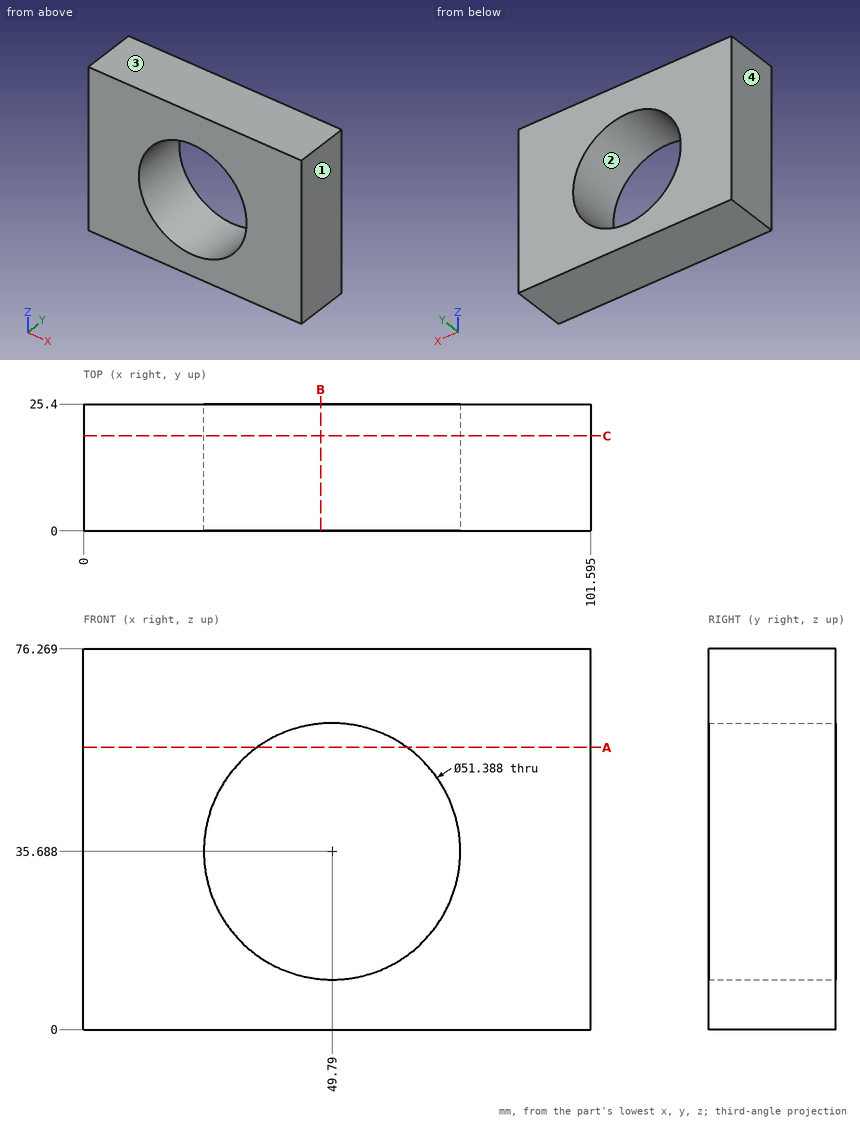
Answer from the drawing. Dimensions are ordinates in mm from the lowest x, y and z of the part. Coordinates: 2 decimals unless noted, no trailing zeros. Order: outer loops, then holes, each group sorted by start corner. A loop starts at its lowest first (then second) coordinate and runs counter-clockwise, first axis right, second up. Notation, with made-up numbers: (67.5, -1.5) -> (108.5, -1.5) arc R22 ccw to (108.5, 20.5) -> close; hole circle Ø8 at (74, 51). An arc over 180 degrees is marked (long way). Answer as a JSON object with one key per item and string values.
1) This flat-tipped pin is pushed along its axis until it touches: pin 1 (4 mm diameter, centred on x = 68, z = 22, fed in from -Y). Where does it stop, or does it pass through?
Model answer:
{"pin 1": "passes through"}
2) A cutting plane is placed at B-B, the plane x = 47.5. Determine the outline of the cut face in (y, z).
Model answer:
{"outline": "(0, 0) -> (25.4, 0) -> (25.4, 10.1) -> (0, 10.1) -> close; (0, 61.28) -> (25.4, 61.28) -> (25.4, 76.27) -> (0, 76.27) -> close"}
3) A cutting plane is placed at C-C, the plane y = 19. Determine the outline of the cut face in (x, z) (1 decimal).
Model answer:
{"outline": "(0, 0) -> (101.6, 0) -> (101.6, 76.3) -> (0, 76.3) -> close; hole circle Ø51.4 at (49.8, 35.7)"}
4) Consider line 1 along X through (y, z) = (9.5, 47) (1 decimal); line 2 along X through (y, z) = (16.5, 30.5) (1 decimal); line 3 along Z through (x, y) = (55.5, 19.5). Determine where each line is inside the solid, lowest interval first. Write a range as from..to.
Model answer:
{"line 1": "x = 0..26.7, 72.9..101.6", "line 2": "x = 0..24.6, 75..101.6", "line 3": "z = 0..10.64, 60.74..76.27"}
5) A cutting plane is placed at A-A, the plane z = 56.5. Determine the outline of the cut face in (x, y) (1 decimal), plus the area to 4 significant figures.
Model answer:
{"outline": "(0, 0) -> (34.7, 0) -> (34.7, 25.4) -> (0, 25.4) -> close; (64.9, 0) -> (101.6, 0) -> (101.6, 25.4) -> (64.9, 25.4) -> close", "area": "1,815 mm²"}
6) The mould has two halves that part along X. Classify the marked faces 1, 2, 3 and 4: released by +X, released by -X, zero draft, split by the parting line, or undercut.
Model answer:
{"face 1": "released by +X", "face 2": "undercut", "face 3": "zero draft", "face 4": "released by -X"}
